Geometry: final body of the model. Coordinates: model frame, mm. Round coordinates to 2 decimals unless told otherwise and drop trailing zeros. Loops run counter-clockwise (first coordinate to the right, second up) from the corner with the lowest first, then second, coordinate; pieces in that order, holes last. Notation, with made-up numbers: (55, 7.5) -> (97, 7.5) arc R30 ccw to (97, 36.5) -> close; hole circle Ø3 at (79, 68). An arc over 180 degrees is marked (long way). Answer in a Markdown table with one row per item.
```python
from build123d import *

# Parameters (mm, degrees)
F0_W        = 21
F0_H        = 260
F1_DEPTH    = 4
F3_DEPTH    = 4.001
F4_T1_DEPTH = 284.4948974279


# Not quite as in the source:
# - a fillet or chamfer that OpenCascade refuses, or shapes differently, is made with other operations: its cross-section is extruded or revolved along the edge and cut away or added


with BuildPart() as f1:
    # F0 (on Top) → F1 (new body)
    with BuildSketch(Plane.XY):
        Rectangle(F0_W, F0_H)
    extrude(amount=F1_DEPTH)

    # F2 (on face) → F3 (cut, through all)
    with BuildSketch(Plane.XY.offset(4)):
        Polygon((10.5, 130), (-10.5, 130), (10.5, 109), align=None)
        Polygon((10.5, -109), (-10.5, -130), (10.5, -130), align=None)
    extrude(amount=-F3_DEPTH, mode=Mode.SUBTRACT)

    # F4: fillet of radius 5 on 1 edges, made by hand

    # F4_s2 → F4_t1 (cut)
    with BuildSketch(Plane.XZ.offset(-142.2474487139)):
        with BuildLine():
            ThreePointArc((-5.6010205144, 4), (-8.7632981746, 2.8729833462), (-10.5, 0))
            Line((-10.5, 0), (-10.5, 4))
            Line((-10.5, 4), (-5.6010205144, 4))
        make_face()
    extrude(amount=F4_T1_DEPTH, mode=Mode.SUBTRACT)


solid = f1.part
```
Item 1: Section query A-A, the plane x = 4.5. Output: boundary loops of the cut face in (y, z), and give its area (3 significant figures).
Ans:
| item | result |
|---|---|
| outline | (-115, 0) -> (115, 0) -> (115, 4) -> (-115, 4) -> close |
| area | 920 mm2 |
Item 2: Section query B-B, the plane y = 91. Output: boundary loops of the cut face in (x, z), and give its area (3 significant figures).
Ans:
| item | result |
|---|---|
| outline | (-10.5, 0) -> (10.5, 0) -> (10.5, 4) -> (-5.6, 4) arc R5 ccw to start |
| area | 79.1 mm2 |
Item 3: Ray query, L1, parallel to Y at x = 6.5, z = 2.9; L2, parallel to X at y = -63, z = 1.6; L3, parallel to X at y = -39.5, z = 1.7. Return the intervals inside material, ascending.
Ans:
| item | result |
|---|---|
| L1 | -113 to 113 |
| L2 | -9.87 to 10.5 |
| L3 | -9.81 to 10.5 |
Item 4: First-contact query: P1, Ø1.5, axis at x = 6.5, z = 2, coming from the +Y side; P2, Ø1, axis at y = 29, z = 2, coming from the -X side; P3, Ø1.5, axis at x = 3, z = 3, coming from the +Y side; P4, Ø1.5, axis at x = 1, y = -101, coming from the -Z side. Flat tips, straight axial feed; report the tip coordinate or a pass-through.
Ans:
| item | result |
|---|---|
| P1 | y = 113.75 |
| P2 | x = -9.93 |
| P3 | y = 117.25 |
| P4 | z = 0 |
